from build123d import *

# Parameters (mm, degrees)
SKETCH1_R           = 9.525
BOSS_EXTRUDE1_DEPTH = 30.01264


with BuildPart() as part:
    # Sketch1 → Boss-Extrude1 (new body)
    with BuildSketch(Plane.XY):
        with Locations(Location((0, 0, 0), (0, 0, 180))):
            Circle(SKETCH1_R)
        Polygon((0, 7.478995387), (-6.477, 3.739497694), (-6.477, -3.739497694), (0, -7.478995387), (6.477, -3.739497694), (6.477, 3.739497694), align=None, mode=Mode.SUBTRACT)
    extrude(amount=BOSS_EXTRUDE1_DEPTH)


solid = part.part
Input: part model. Units: mm. Frame: model coordinates. A direction names the side the tool comes from. Give positions to 0.01 mm unless a question says otherwise; leave off trailing zeros. Order: outer loops, then holes, each group sorted by start corner. A loop starts at its lowest first (then second) coordinate and runs counter-clockwise, first axis right, second up. Notation, with made-up numbers: (-13.5, 27.25) -> (16.5, 27.25) arc R16 ccw to (16.5, 45.25) -> close; hole circle Ø3 at (-26.75, 32.25). An arc over 180 degrees is marked (long way). Use one line per item in the form item = value.
1) Line query: probe 1 along X at (y, z) = (7, 16); probe 2 along Y at (x, z) = (-1.75, 13.5); probe 3 along X at (y, z) = (6, 3). Output: solid intervals per line, ascending.
Response values:
probe_1 = -6.46 to -0.83, 0.83 to 6.46
probe_2 = -9.36 to -6.47, 6.47 to 9.36
probe_3 = -7.4 to -2.56, 2.56 to 7.4
2) Section B-B, the plane x = -2.5. Return loops of the section in (y, z), and give its area (3 significant figures).
Response values:
outline = (-9.19, 0) -> (-6.04, 0) -> (-6.04, 30.01) -> (-9.19, 30.01) -> close; (6.04, 0) -> (9.19, 0) -> (9.19, 30.01) -> (6.04, 30.01) -> close
area = 189 mm^2
3) First-contact query: pin 1 Ø8 at (y, z) = (-1.5, 11.5) entering from +X (3 decimals); pin 2 Ø1 at (x, z) = (5, 10) entering from -Y (3 decimals); pin 3 Ø10 at (x, z) = (-7, 9.5) entering from +Y; pin 4 Ø3 at (y, z) = (-2, 14) entering from -X. Flat tips, straight axial feed; report the tip coordinate or a pass-through.
Response values:
pin_1 = 9.525
pin_2 = -8.395
pin_3 = 9.31
pin_4 = -9.51
4) Section C-C, the plane y = 0. Return loops of the section in (x, z) (3 decimals), and give its area (3 significant figures).
Response values:
outline = (-9.525, 0) -> (-6.477, 0) -> (-6.477, 30.013) -> (-9.525, 30.013) -> close; (6.477, 0) -> (9.525, 0) -> (9.525, 30.013) -> (6.477, 30.013) -> close
area = 183 mm^2
5) Mould query, pull axis Y, two halves, no side actions, for faces 3 (the cylindrical face through (2.06, 9.3, 14.8)), 4 (the flat face through (-3.193, 5.635, 14.796)), 5 (the flat face through (2.3, -6.5, 0)). Classes: pulls with the +Y half, pulls with the -Y half, needs draft (parallel to the pull), parting line crosses it, or undercut.
Response values:
face_3 = parting line crosses it
face_4 = undercut
face_5 = needs draft
6) Reachability of faces 1 (the flat face through (2.3, -6.5, 30.013)), 2 (the flat face through (-6.477, 0, 15)) from +Z, -Z, +X, -X, +Y, -Y: full face, straight path, thin tool, end or side. Return the list, or none.
Response values:
face_1 = +Z, +X, -X, +Y, -Y
face_2 = +Z, -Z
